from build123d import *

# Parameters (mm, degrees)
F0_W     = 12.7
F0_H     = 5.08
F1_DEPTH = 12.7
F3_DEPTH = 3.81
F5_DEPTH = 3.81
F7_DEPTH = 3.81
F9_DEPTH = 5.08


with BuildPart() as f1:
    # F0 (on Front) → F1 (new body)
    with BuildSketch(Plane.XZ):
        with Locations((-6.35, 2.54)):
            Rectangle(F0_W, F0_H)
        Polygon((0, 5.08), (0, 0), (12.7, 0), (12.7, 25.4), (0, 25.4), align=None)
    extrude(amount=F1_DEPTH)

    # F2 (on face) → F3 (join)
    with BuildSketch(Plane(origin=(0, 0, 0), x_dir=(1, 0, 0), z_dir=(0, 0, -1))):
        Polygon((-1.905, 8.255), (-1.905, 7.3025), (0, 6.35), (1.905, 7.3025), (1.905, 8.255), align=None)
        Polygon((0, 6.35), (-1.905, 7.3025), (-1.905, 5.3975), align=None)
        Polygon((1.905, 7.3025), (0, 6.35), (1.905, 5.3975), align=None)
        Polygon((1.905, 5.3975), (0, 6.35), (-1.905, 5.3975), (-1.905, 4.445), (1.905, 4.445), align=None)
    extrude(amount=F3_DEPTH)

    # F4 (on face) → F5 (join)
    with BuildSketch(Plane.XZ.offset(8.255)):
        Polygon((1.905, 0), (-1.905, 0), (-24.493341372, -11.6158010512), (-22.7509712143, -15.004052257), (-1.905, -3.81), (1.905, -3.81), (25.7752793361, -12.4915761481), (27.0466815017, -8.8999697479), align=None)
    extrude(amount=-F5_DEPTH)

    # F6 (on face) → F7 (join)
    with BuildSketch(Plane.XZ.offset(8.255)):
        Polygon((-23.3987490657, 10.877285878), (-24.493341372, -11.6158010512), (-20.5809258805, -9.6038852921), (-19.5932523682, 10.6920970944), align=None)
    extrude(amount=-F7_DEPTH)

    # F8 (on face) → F9 (join)
    with BuildSketch(Plane(origin=(0, -4.445, 0), x_dir=(-1, 0, 0), z_dir=(0, 1, 0))):
        with BuildLine():
            ThreePointArc((-22.7051897472, -10.0496184245), (-22.9990213636, -9.0331729319), (-23.7898736732, -8.3302852576))
            Line((-23.7898736732, -8.3302852576), (-24.6101897472, -10.0496184245))
            Line((-24.6101897472, -10.0496184245), (-22.8873458267, -10.8625352872))
            ThreePointArc((-22.8873458267, -10.8625352872), (-22.7512864861, -10.4661561368), (-22.7051897472, -10.0496184245))
        make_face()
        with BuildLine():
            Line((-24.6101897472, -10.0496184245), (-23.7898736732, -8.3302852576))
            ThreePointArc((-23.7898736732, -8.3302852576), (-25.2497495627, -8.2551858561), (-26.3330336677, -9.2367015618))
            Line((-26.3330336677, -9.2367015618), (-24.6101897472, -10.0496184245))
        make_face()
        with BuildLine():
            Line((-22.8873458267, -10.8625352872), (-24.6101897472, -10.0496184245))
            Line((-24.6101897472, -10.0496184245), (-25.4305058212, -11.7689515914))
            ThreePointArc((-25.4305058212, -11.7689515914), (-23.9706299318, -11.8440509929), (-22.8873458267, -10.8625352872))
        make_face()
        with BuildLine():
            Line((-25.4305058212, -11.7689515914), (-24.6101897472, -10.0496184245))
            Line((-24.6101897472, -10.0496184245), (-26.3330336677, -9.2367015618))
            ThreePointArc((-26.3330336677, -9.2367015618), (-26.4046223156, -10.68917824), (-25.4305058212, -11.7689515914))
        make_face()
        with BuildLine():
            ThreePointArc((22.5584327346, -10.6207959991), (21.9501618456, -10.5111051642), (21.338789094, -10.6019286869))
            Line((21.338789094, -10.6019286869), (21.9206959191, -12.4158772658))
            Line((21.9206959191, -12.4158772658), (23.7397587132, -11.8501604187))
            ThreePointArc((23.7397587132, -11.8501604187), (23.4578969896, -11.2906937835), (23.009799723, -10.8529064074))
            Line((23.009799723, -10.8529064074), (22.5584327346, -10.6207959991))
        make_face()
        with BuildLine():
            Line((21.9206959191, -12.4158772658), (21.338789094, -10.6019286869))
            ThreePointArc((21.338789094, -10.6019286869), (20.2304694068, -11.537151292), (20.101633125, -12.9815941129))
            Line((20.101633125, -12.9815941129), (21.9206959191, -12.4158772658))
        make_face()
        with BuildLine():
            Line((23.7397587132, -11.8501604187), (21.9206959191, -12.4158772658))
            Line((21.9206959191, -12.4158772658), (22.5026027442, -14.2298258447))
            ThreePointArc((22.5026027442, -14.2298258447), (23.4597796566, -13.5384841646), (23.8256959191, -12.4158772658))
            ThreePointArc((23.8256959191, -12.4158772658), (23.8040890834, -12.1297738079), (23.7397587132, -11.8501604187))
        make_face()
        with BuildLine():
            Line((22.5026027442, -14.2298258447), (21.9206959191, -12.4158772658))
            Line((21.9206959191, -12.4158772658), (20.101633125, -12.9815941129))
            ThreePointArc((20.101633125, -12.9815941129), (21.0419699453, -14.1061037782), (22.5026027442, -14.2298258447))
        make_face()
        with BuildLine():
            ThreePointArc((23.009799723, -10.8529064074), (22.7918809979, -10.7217516629), (22.5584327346, -10.6207959991))
            Line((22.5584327346, -10.6207959991), (23.009799723, -10.8529064074))
        make_face()
    extrude(amount=F9_DEPTH)


solid = f1.part
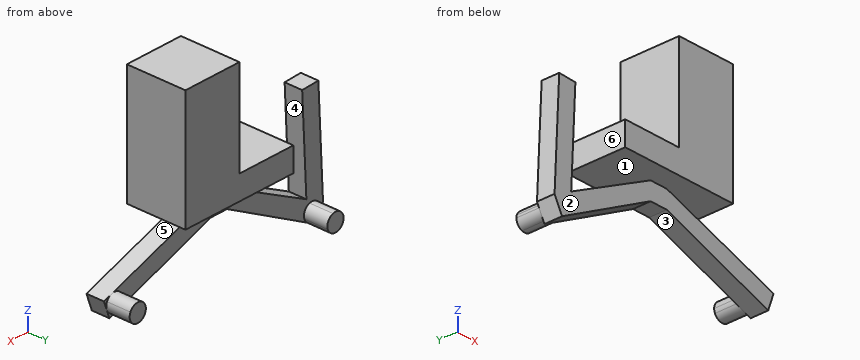
The model under review builds one solid part; all positions refer to its coordinate system, in mm. Face numbers are marked on the shaded views. A direction names the side the tool comes from. Coordinates: 2 decimals unless noted, no trailing zeros. Loops run counter-clockwise (first coordinate to the right, second up) from the corner with the lowest first, then second, coordinate; pieces in that order, holes last. Notation, with made-up numbers: (77, 50.5) -> (125, 50.5) arc R29 ccw to (125, 74.5) -> close; hole circle Ø8 at (68, 77.5). An arc over 180 degrees is marked (long way). Use a Markdown table: item, result. Add a question column.
1. Clearance check with flat-ended pins moving along their axes: pin 1 Ø6 at (y, z) = (-4.5, 14) entering from +X; pin 2 Ø20.5 at (x, z) = (-2.5, -2.5) entering from +Y; pin 3 Ø6 at (y, z) = (-3.5, 4) entering from -X. State where each tip first meets the part, or that it passes through.
2. Add section C-C on z = 8. Write out the cut boundary in (x, y) (3 decimals), plus the area to 3 significant figures.
3. Draft analysis for pull direction Z (two halves, no side actions). For the marked faces 1, 2 and 3, state which applies: pulls with the +Z half, pulls with the -Z half, needs draft (parallel to the pull), parting line crosses it, or undercut.
4. Add section B-B on x = -6. Write out the cut boundary in (y, z) (3 decimals).
5. Machinability: for the marked faces 4, 5 and 6, which of the approach directions +Z, -Z, +X, -X, +Y, -Y give a long, thin tool a straight path to every point of the face, cutting with its end or side? Answer none if there is none.
6. Add section A-A on y = -2.75. Write out the cut boundary in (x, z) (1 decimal).
7. To check wall thickness, follow line 1 (X direction, y = -10.25, z = 4.5); line 2 (Z direction, x = -4, y = -11.5); line 3 (Y direction, x = -19, z = -11) (3 decimals). State the ranges of each line that lie inside material, in increasing order.
8. Add section D-D on y = -10. Write out the cut boundary in (x, z).
Returned:
| question | item | result |
|---|---|---|
| 1 | pin 1 | stops at x = 12.7 |
| 1 | pin 2 | stops at y = 0 |
| 1 | pin 3 | stops at x = -23.87 |
| 2 | outline | (-23.539, -8.255) -> (-19.724, -8.255) -> (-19.724, -4.445) -> (-23.539, -4.445) -> close; (0, -12.7) -> (12.7, -12.7) -> (12.7, 0) -> (0, 0) -> close |
| 2 | area | 176 mm² |
| 3 | face 1 | undercut |
| 3 | face 2 | needs draft |
| 3 | face 3 | pulls with the -Z half |
| 4 | outline | (-12.7, 0) -> (0, 0) -> (0, 5.08) -> (-12.7, 5.08) -> close; (-8.255, -6.009) -> (-4.445, -6.009) -> (-4.445, -2.106) -> (-8.255, -2.106) -> close |
| 5 | face 4 | +Y, -Y |
| 5 | face 5 | +X, +Y, -Y |
| 5 | face 6 | +Z, +Y, -Y |
| 6 | outline | circle Ø3.8 at (-21.9, -12.4); (-12.7, 0) -> (12.7, 0) -> (12.7, 25.4) -> (0, 25.4) -> (0, 5.1) -> (-12.7, 5.1) -> close; circle Ø3.8 at (24.6, -10) |
| 7 | line 1 | x = -12.7 to 12.7 |
| 7 | line 2 | z = 0 to 5.08 |
| 7 | line 3 | y = -8.255 to -4.445 |
| 8 | outline | (-12.7, 0) -> (12.7, 0) -> (12.7, 25.4) -> (0, 25.4) -> (0, 5.08) -> (-12.7, 5.08) -> close |
